Autodesk Inventor part; units mm, degrees
ref_plane "Plan YZ" through (0, 0, 0) normal (1, 0, 0) x (0, 1, 0)
ref_plane "Plan XZ" through (0, 0, 0) normal (0, 1, 0) x (-1, 0, 0)
ref_plane "Plan XY" through (0, 0, 0) normal (0, 0, 1) x (1, 0, 0)
sketch "Esquisse1" plane through (0, 0, 0) normal (0, 0, 1) x (1, 0, 0)
  line L0 (0, -58.1) -> (0, 58.1) construction
  line L1 (-112, 0) -> (112, 0) construction
  line L2 (-75, 37.5) -> (-75, 41.5)
  line L3 (-75, 41.5) -> (-60, 41.5)
  line L4 (-60, 41.5) -> (-60, 37.5)
  line L5 (-30, 37.5) -> (-30, 41.5)
  line L6 (-30, 41.5) -> (-15, 41.5)
  line L7 (-15, 41.5) -> (-15, 37.5)
  line L8 (15, 37.5) -> (15, 41.5)
  line L9 (15, 41.5) -> (30, 41.5)
  line L10 (30, 41.5) -> (30, 37.5)
  line L11 (60, 37.5) -> (60, 41.5)
  line L12 (60, 41.5) -> (75, 41.5)
  line L13 (75, 41.5) -> (75, 37.5)
  line L14 (-60, 37.5) -> (-30, 37.5)
  line L15 (-15, 37.5) -> (15, 37.5)
  line L16 (30, 37.5) -> (60, 37.5)
  line L17 (-75, 37.5) -> (-80, 37.5)
  line L18 (75, 37.5) -> (80, 37.5)
  line L19 (-75, -37.5) -> (-75, -41.5)
  line L20 (-75, -41.5) -> (-60, -41.5)
  line L21 (-60, -41.5) -> (-60, -37.5)
  line L22 (-30, -37.5) -> (-30, -41.5)
  line L23 (-30, -41.5) -> (-15, -41.5)
  line L24 (-15, -41.5) -> (-15, -37.5)
  line L25 (15, -37.5) -> (15, -41.5)
  line L26 (15, -41.5) -> (30, -41.5)
  line L27 (30, -41.5) -> (30, -37.5)
  line L28 (60, -37.5) -> (60, -41.5)
  line L29 (60, -41.5) -> (75, -41.5)
  line L30 (75, -41.5) -> (75, -37.5)
  line L31 (-60, -37.5) -> (-30, -37.5)
  line L32 (-15, -37.5) -> (15, -37.5)
  line L33 (30, -37.5) -> (60, -37.5)
  line L34 (-75, -37.5) -> (-80, -37.5)
  line L35 (75, -37.5) -> (80, -37.5)
  line L36 (80, -37.5) -> (80, 37.5)
  line L37 (-80, 37.5) -> (-80, -37.5)
  dimension "d2" = 15
  dimension "d8" = 45
  dimension "d13" = 5
  dimension "d14" = 5
  dimension "d15" = 75
  dimension "d16" = 4
  dimension "d17" = 160
extrude "Extrusion1" add sketch "Esquisse1" along normal blind 4
sketch "Esquisse6" plane through (0, 0, 4) normal (0, 0, 1) x (1, 0, 0)
  line L0 (0, -58.1) -> (0, 58.1) construction
  line L1 (-112, 0) -> (112, 0) construction
  point P0 (0, 0)
  point P1 (-75, 37.5)
  point P2 (-60, 37.5)
  point P3 (-30, 37.5)
  point P4 (-15, 37.5)
  point P5 (15, 37.5)
  point P6 (75, 37.5)
  point P7 (30, 37.5)
  point P8 (60, 37.5)
  point P9 (-75, -37.5)
  point P10 (-60, -37.5)
  point P11 (-30, -37.5)
  point P12 (-15, -37.5)
  point P13 (15, -37.5)
  point P14 (75, -37.5)
  point P15 (30, -37.5)
  point P16 (60, -37.5)
hole "Perçage1" at (-75, 37.5, 4) at (-60, 37.5, 4) at (-30, 37.5, 4) at (-15, 37.5, 4) at (15, 37.5, 4) at (75, 37.5, 4) at (30, 37.5, 4) at (60, 37.5, 4) at (60, -37.5, 4) at (30, -37.5, 4) at (75, -37.5, 4) at (15, -37.5, 4) at (-15, -37.5, 4) at (-30, -37.5, 4) at (-60, -37.5, 4) at (-75, -37.5, 4) direction (0, 0, -1) diameter 1 end through all
chamfer "Chanfrein1" distance 1 angle 45 16 edges at (75, 41.5, 2) (60, 41.5, 2) (15, 41.5, 2) (-30, 41.5, 2) (-75, 41.5, 2) (30, 41.5, 2) (-15, 41.5, 2) (-60, 41.5, 2) (-60, -41.5, 2) (-15, -41.5, 2) (30, -41.5, 2) (75, -41.5, 2) (60, -41.5, 2) (-75, -41.5, 2) (-30, -41.5, 2) (15, -41.5, 2)
properties part number "P1704_005" material "Plastique PMMA"
Build history of the part. All positions in model axes, mm. A direction names the side the tool comes from. Round coordinates to 2 decimals unless told otherwise and drop trailing zeros. Write each loop counter-clockwise with the first axis right and the second up, starting at its lowest first coordinate (ties: lowest second). Pieces come first, ordered by that corner, then holes. Notation, with made-up numbers: (69.25, 17) -> (104.25, 17) arc R29 ccw to (104.25, 51) -> close; hole circle Ø2 at (-32.5, 41.5). An arc over 180 degrees is marked (long way). Use one line per item in the form item = value.
Q1. Band-saw the part on A-A, the plane x = -58. Write the cut outline in (y, z).
Conclusion:
outline = (-37.5, 0) -> (37.5, 0) -> (37.5, 4) -> (-37.5, 4) -> close
Q2. Tool access for faces 1 (the flat face through (0, 37.5, 2)), 2 (the flat face through (-45, -37.5, 2)), 3 (the flat face through (-78, 37.5, 2)): list every direction of +Z, -Z, +X, -X, +Y, -Y with a clear straight run to the whole face (end or side of a thin tool).
Conclusion:
face_1 = +Z, -Z, +Y
face_2 = +Z, -Z, -Y
face_3 = +Z, -Z, -X, +Y
Q3. Two-plate mould, pull along X, no slides. Class faces 4 (the flat face through (22, 41.5, 2)), 5 (the flat face through (45, 37.5, 2)): released by +X, released by -X, zero draft, split by the parting line, or undercut.
Conclusion:
face_4 = zero draft
face_5 = undercut
Q4. Drop flat-ended pins along their axis: P1, Ø2, axis at x = 76.5, z = 2.5, coming from the -Y side; P2, Ø0.8, axis at y = -39.5, z = 2.5, coming from the +X side; P3, Ø2, axis at x = 42, z = 3, coming from the +Y side. Give the stop position or say it passes through.
Conclusion:
P1 = -37.5
P2 = 75
P3 = 37.5
Q5. Drill centre line: L1, parallel to Y at x = -52, z = 1.25. Where is it in solid material? Low to high.
Conclusion:
L1 = -37.5 to 37.5
